Build history of the part. All positions in model axes, mm. Round coordinates to 2 decimals unless told otherwise and drop trailing zeros. Order: outer loops, then holes, each group sorted by start corner. A loop starts at its lowest first (then second) coordinate and runs counter-clockwise, first axis right, second up. Notation, with made-up numbers: M 0.5,2.5 L 11.5,2.5 A25 cw 11.5,14.5 Z; hole C 87.5,80.5 d1. An arc over 180 degrees is marked long. One line per item, written item: value. Start each with the question number.
Item 1: Band-saw the part on C-C, the plane y = -22. Write the cut outline in (x, z), then the cut area to 3 significant figures.
Item 2: Two-plate mould, pull along X, no slides. Class faces 1 (the flat face through (0, 30, 7)), 2 (the cylindrical face through (-12.33, 24.48, 7.54)), 3 (the cylindrical face through (18, 29, 8)): +X half, -X half, draft (parallel to the pull), parting line (faces both ways), or undercut.
Item 3: Probe L1, parallel to Y at x = -12, z = 6.8; L2, parallel to X at y = -22, z = 6.45; L3, parallel to X at y = 20, z = 9.6. List the from-to ranges inside material, lowest first.
Item 4: Band-saw the part on B-B, the plane x = 12. Write the cut outline in (y, z), then the cut area to 3 significant figures.
Item 5: Pin check, flat tip, straight feed: pin 1 (4 mm diameter, centred on x = 12, y = -22, fed in from +Z). Stop position of the tip, or through.
Item 6: Band-saw the part on A-A, the plane z = 8.35. Write the cut outline in (x, y).
```python
from build123d import *

# Parameters (mm, degrees)
SKETCH011_W     = 40
SKETCH011_H     = 60
PAD003_DEPTH    = 5
SKETCH017_R     = 2.5
POCKET009_DEPTH = 5
FILLET004_R     = 5


with BuildPart() as part:
    # Sketch011 → Pad003 (new body)
    with BuildSketch(Plane.XY):
        Rectangle(SKETCH011_W, SKETCH011_H)
    extrude(amount=PAD003_DEPTH)

    # Sketch017 (on Face6 of Pad003) → Pocket009 (cut)
    with BuildSketch(Plane.XY.offset(5)):
        with Locations((-12, 22)):
            Circle(SKETCH017_R)
        with Locations((12, 22)):
            Circle(SKETCH017_R)
    pocket009 = extrude(amount=-POCKET009_DEPTH, mode=Mode.SUBTRACT)

    # Mirrored001: Pocket009 across XZ
    add(pocket009.mirror(Plane.XZ), mode=Mode.SUBTRACT)

    # Fillet004
    fillet004_edges = [part.edges().sort_by_distance(p)[0] for p in [
        (20, 30, 2.5),
        (-20, 30, 2.5),
        (-20, -30, 2.5),
        (20, -30, 2.5),
    ]]
    fillet(fillet004_edges, radius=FILLET004_R)


with BuildPart() as part_1:
    # Body003 placement: moved
    add(part.part.moved(Location((0, 0, 5))))


solid = part_1.part
```
Output:
1. outline: M -20,5 L -14.5,5 L -14.5,10 L -20,10 Z; M -9.5,5 L 9.5,5 L 9.5,10 L -9.5,10 Z; M 14.5,5 L 20,5 L 20,10 L 14.5,10 Z
1. area: 150 mm²
2. face 1: draft
2. face 2: undercut
2. face 3: +X half
3. L1: y = -30 to -24.5, -19.5 to 19.5, 24.5 to 30
3. L2: x = -20 to -14.5, -9.5 to 9.5, 14.5 to 20
3. L3: x = -20 to -13.5, -10.5 to 10.5, 13.5 to 20
4. outline: M -30,5 L -24.5,5 L -24.5,10 L -30,10 Z; M -19.5,5 L 19.5,5 L 19.5,10 L -19.5,10 Z; M 24.5,5 L 30,5 L 30,10 L 24.5,10 Z
4. area: 250 mm²
5. pin 1: passes through
6. outline: M -20,-25 A5 ccw -15,-30 L 15,-30 A5 ccw 20,-25 L 20,25 A5 ccw 15,30 L -15,30 A5 ccw -20,25 Z; hole C -12,-22 d5; hole C -12,22 d5; hole C 12,-22 d5; hole C 12,22 d5
